The model under review builds one solid part; all positions refer to its coordinate system, in mm. Give positions to 0.01 mm unless a question says otherwise; leave off trailing zeros. Loops run counter-clockwise (first coordinate to the right, second up) from the corner with the lowest first, then second, coordinate; pieces in that order, holes last. Notation, with made-up numbers: M 11,15 L 45,15 A11 cw 45,19 Z; hole C 47.5,4.25 d2. An arc over 180 degrees is marked long. Return JSON: item names as keys, results as strings. Group by question number.
```python
from build123d import *

# Parameters (mm, degrees)
F0_R     = 3.35
F1_DEPTH = 100


with BuildPart() as f1:
    # F0 (on Top) → F1 (new body)
    with BuildSketch(Plane.XY):
        with BuildLine():
            Line((20, -15.994185), (20, -5.1))
            ThreePointArc((20, -5.1), (19.707107, -4.392893), (19, -4.1))
            Line((19, -4.1), (16.35, -4.1))
            ThreePointArc((16.35, -4.1), (15.642893, -4.392893), (15.35, -5.1))
            Line((15.35, -5.1), (15.35, -6.1))
            ThreePointArc((15.35, -6.1), (15.642893, -6.807107), (16.35, -7.1))
            Line((16.35, -7.1), (17.85, -7.1))
            ThreePointArc((17.85, -7.1), (18.203553, -7.246447), (18.35, -7.6))
            ThreePointArc((18.35, -7.6), (17.617767, -9.367767), (15.85, -10.1))
            Line((15.85, -10.1), (13.993362, -10.1))
            ThreePointArc((13.993362, -10.1), (13.036864, -9.909786), (12.225917, -9.368088))
            Line((12.225917, -9.368088), (8.332554, -5.476141))
            ThreePointArc((8.332554, -5.476141), (7.790388, -4.664971), (7.6, -3.708053))
            Line((7.6, -3.708053), (7.6, 3.708053))
            ThreePointArc((7.6, 3.708053), (7.790388, 4.664971), (8.332554, 5.476141))
            Line((8.332554, 5.476141), (12.225917, 9.368088))
            ThreePointArc((12.225917, 9.368088), (13.036864, 9.909786), (13.993362, 10.1))
            Line((13.993362, 10.1), (15.85, 10.1))
            ThreePointArc((15.85, 10.1), (17.617767, 9.367767), (18.35, 7.6))
            ThreePointArc((18.35, 7.6), (18.203553, 7.246447), (17.85, 7.1))
            Line((17.85, 7.1), (16.35, 7.1))
            ThreePointArc((16.35, 7.1), (15.642893, 6.807107), (15.35, 6.1))
            Line((15.35, 6.1), (15.35, 5.1))
            ThreePointArc((15.35, 5.1), (15.642893, 4.392893), (16.35, 4.1))
            Line((16.35, 4.1), (19, 4.1))
            ThreePointArc((19, 4.1), (19.707107, 4.392893), (20, 5.1))
            Line((20, 5.1), (20, 16.004817))
            ThreePointArc((20, 16.004817), (18.827561, 18.834111), (15.997549, 20.004817))
            Line((15.997549, 20.004817), (5.10727, 19.998145))
            ThreePointArc((5.10727, 19.998145), (4.400057, 19.705509), (4.106906, 18.998508))
            Line((4.106906, 18.998508), (4.105943, 16.348509))
            ThreePointArc((4.105943, 16.348509), (4.398579, 15.641295), (5.105579, 15.348145))
            Line((5.105579, 15.348145), (6.105579, 15.347782))
            ThreePointArc((6.105579, 15.347782), (6.812793, 15.640418), (7.105943, 16.347418))
            Line((7.105943, 16.347418), (7.106488, 17.847418))
            ThreePointArc((7.106488, 17.847418), (7.253063, 18.200918), (7.60667, 18.347236))
            ThreePointArc((7.60667, 18.347236), (9.374171, 17.614361), (10.105761, 15.846328))
            Line((10.105761, 15.846328), (10.105086, 13.98969))
            ThreePointArc((10.105086, 13.98969), (9.914524, 13.03326), (9.372532, 12.222511))
            Line((9.372532, 12.222511), (5.479169, 8.330563))
            ThreePointArc((5.479169, 8.330563), (4.667803, 7.788692), (3.710815, 7.598652))
            Line((3.710815, 7.598652), (-3.710815, 7.598652))
            ThreePointArc((-3.710815, 7.598652), (-4.667803, 7.788692), (-5.479169, 8.330563))
            Line((-5.479169, 8.330563), (-9.372532, 12.222511))
            ThreePointArc((-9.372532, 12.222511), (-9.914524, 13.03326), (-10.105086, 13.98969))
            Line((-10.105086, 13.98969), (-10.105761, 15.846328))
            ThreePointArc((-10.105761, 15.846328), (-9.374171, 17.614361), (-7.60667, 18.347236))
            ThreePointArc((-7.60667, 18.347236), (-7.253063, 18.200918), (-7.106488, 17.847418))
            Line((-7.106488, 17.847418), (-7.105943, 16.347418))
            ThreePointArc((-7.105943, 16.347418), (-6.812793, 15.640418), (-6.105579, 15.347782))
            Line((-6.105579, 15.347782), (-5.105579, 15.348145))
            ThreePointArc((-5.105579, 15.348145), (-4.398579, 15.641295), (-4.105943, 16.348509))
            Line((-4.105943, 16.348509), (-4.106906, 18.998508))
            ThreePointArc((-4.106906, 18.998508), (-4.400057, 19.705509), (-5.10727, 19.998145))
            Line((-5.10727, 19.998145), (-16.001454, 19.994185))
            ThreePointArc((-16.001454, 19.994185), (-18.828941, 18.822098), (-20, 15.994185))
            Line((-20, 15.994185), (-20, 5.1))
            ThreePointArc((-20, 5.1), (-19.707107, 4.392893), (-19, 4.1))
            Line((-19, 4.1), (-16.35, 4.1))
            ThreePointArc((-16.35, 4.1), (-15.642893, 4.392893), (-15.35, 5.1))
            Line((-15.35, 5.1), (-15.35, 6.1))
            ThreePointArc((-15.35, 6.1), (-15.642893, 6.807107), (-16.35, 7.1))
            Line((-16.35, 7.1), (-17.85, 7.1))
            ThreePointArc((-17.85, 7.1), (-18.203553, 7.246447), (-18.35, 7.6))
            ThreePointArc((-18.35, 7.6), (-17.617767, 9.367767), (-15.85, 10.1))
            Line((-15.85, 10.1), (-13.993362, 10.1))
            ThreePointArc((-13.993362, 10.1), (-13.036864, 9.909786), (-12.225917, 9.368088))
            Line((-12.225917, 9.368088), (-8.332554, 5.476141))
            ThreePointArc((-8.332554, 5.476141), (-7.790388, 4.664971), (-7.6, 3.708053))
            Line((-7.6, 3.708053), (-7.6, -3.708053))
            ThreePointArc((-7.6, -3.708053), (-7.790388, -4.664971), (-8.332554, -5.476141))
            Line((-8.332554, -5.476141), (-12.225917, -9.368088))
            ThreePointArc((-12.225917, -9.368088), (-13.036864, -9.909786), (-13.993362, -10.1))
            Line((-13.993362, -10.1), (-15.85, -10.1))
            ThreePointArc((-15.85, -10.1), (-17.617767, -9.367767), (-18.35, -7.6))
            ThreePointArc((-18.35, -7.6), (-18.203553, -7.246447), (-17.85, -7.1))
            Line((-17.85, -7.1), (-16.35, -7.1))
            ThreePointArc((-16.35, -7.1), (-15.642893, -6.807107), (-15.35, -6.1))
            Line((-15.35, -6.1), (-15.35, -5.1))
            ThreePointArc((-15.35, -5.1), (-15.642893, -4.392893), (-16.35, -4.1))
            Line((-16.35, -4.1), (-19, -4.1))
            ThreePointArc((-19, -4.1), (-19.707107, -4.392893), (-20, -5.1))
            Line((-20, -5.1), (-20, -15.994185))
            ThreePointArc((-20, -15.994185), (-18.828941, -18.822098), (-16.001454, -19.994185))
            Line((-16.001454, -19.994185), (-5.10727, -19.998145))
            ThreePointArc((-5.10727, -19.998145), (-4.400057, -19.705509), (-4.106906, -18.998508))
            Line((-4.106906, -18.998508), (-4.105943, -16.348509))
            ThreePointArc((-4.105943, -16.348509), (-4.398579, -15.641295), (-5.105579, -15.348145))
            Line((-5.105579, -15.348145), (-6.105579, -15.347782))
            ThreePointArc((-6.105579, -15.347782), (-6.812793, -15.640418), (-7.105943, -16.347418))
            Line((-7.105943, -16.347418), (-7.106488, -17.847418))
            ThreePointArc((-7.106488, -17.847418), (-7.253063, -18.200918), (-7.60667, -18.347236))
            ThreePointArc((-7.60667, -18.347236), (-9.374171, -17.614361), (-10.105761, -15.846328))
            Line((-10.105761, -15.846328), (-10.105086, -13.98969))
            ThreePointArc((-10.105086, -13.98969), (-9.914524, -13.03326), (-9.372532, -12.222511))
            Line((-9.372532, -12.222511), (-5.479169, -8.330563))
            ThreePointArc((-5.479169, -8.330563), (-4.667803, -7.788692), (-3.710815, -7.598652))
            Line((-3.710815, -7.598652), (3.710815, -7.598652))
            ThreePointArc((3.710815, -7.598652), (4.667803, -7.788692), (5.479169, -8.330563))
            Line((5.479169, -8.330563), (9.372532, -12.222511))
            ThreePointArc((9.372532, -12.222511), (9.914524, -13.03326), (10.105086, -13.98969))
            Line((10.105086, -13.98969), (10.105761, -15.846328))
            ThreePointArc((10.105761, -15.846328), (9.374171, -17.614361), (7.60667, -18.347236))
            ThreePointArc((7.60667, -18.347236), (7.253063, -18.200918), (7.106488, -17.847418))
            Line((7.106488, -17.847418), (7.105943, -16.347418))
            ThreePointArc((7.105943, -16.347418), (6.812793, -15.640418), (6.105579, -15.347782))
            Line((6.105579, -15.347782), (5.105579, -15.348145))
            ThreePointArc((5.105579, -15.348145), (4.398579, -15.641295), (4.105943, -16.348509))
            Line((4.105943, -16.348509), (4.106906, -18.998508))
            ThreePointArc((4.106906, -18.998508), (4.400057, -19.705509), (5.10727, -19.998145))
            Line((5.10727, -19.998145), (16.001454, -19.994185))
            ThreePointArc((16.001454, -19.994185), (18.828941, -18.822098), (20, -15.994185))
        make_face()
        with BuildLine():
            ThreePointArc((-16.002998, -18.346327), (-17.664699, -17.658028), (-18.352998, -15.996327))
            Line((-18.352998, -15.996327), (-18.352998, -12.544276))
            Line((-18.352998, -12.544276), (-12.548836, -12.544276))
            Line((-12.548836, -12.544276), (-12.548836, -18.346327))
            Line((-12.548836, -18.346327), (-16.002998, -18.346327))
        make_face(mode=Mode.SUBTRACT)
        with BuildLine():
            ThreePointArc((18.352998, -15.996327), (17.664699, -17.658028), (16.002998, -18.346327))
            Line((16.002998, -18.346327), (12.548836, -18.346327))
            Line((12.548836, -18.346327), (12.548836, -12.544276))
            Line((12.548836, -12.544276), (18.352998, -12.544276))
            Line((18.352998, -12.544276), (18.352998, -15.996327))
        make_face(mode=Mode.SUBTRACT)
        Circle(F0_R, mode=Mode.SUBTRACT)
        with BuildLine():
            Line((-16.002998, 18.346327), (-12.548836, 18.346327))
            Line((-12.548836, 18.346327), (-12.548836, 12.544276))
            Line((-12.548836, 12.544276), (-18.352998, 12.544276))
            Line((-18.352998, 12.544276), (-18.352998, 15.996327))
            ThreePointArc((-18.352998, 15.996327), (-17.664699, 17.658028), (-16.002998, 18.346327))
        make_face(mode=Mode.SUBTRACT)
        with BuildLine():
            Line((12.548836, 18.346327), (16.002998, 18.346327))
            ThreePointArc((16.002998, 18.346327), (17.664699, 17.658028), (18.352998, 15.996327))
            Line((18.352998, 15.996327), (18.352998, 12.544276))
            Line((18.352998, 12.544276), (12.548836, 12.544276))
            Line((12.548836, 12.544276), (12.548836, 18.346327))
        make_face(mode=Mode.SUBTRACT)
    extrude(amount=F1_DEPTH)


solid = f1.part
```
(1) Mouldability with a two-part tool opening along X and no side actions: class faces 1 (the flat face through (-2, 3, 0)), 2 (the flat face through (-7.6, 0, 49)), 3 (the flat face through (18.353, 14, 49)) as released by +X, released by -X, zero draft, split by the parting line, or undercut.
(2) Add section A-A (x = 0). Write out the cut boundary in (y, z), and give its area (3 significant figures).
(3) For probe 1 along Y at (x, z) = (5.5, 83); probe 2 along X at (y, z) = (-5.5, 50); probe 3 along Y at (x, z) = (0, 24), list the stretches that pass through material, from the lowest coordinate up.
(4) Add section C-C (z = 16.5). Count the separate pieces of the cut face and the enclosed holes in it, and give its area (3 significant figures).
(5) For pin 1 (3.5 mm diameter, centred on x = -1, z = 41.5, fed in from -Y); pin 2 (0.8 mm diameter, centred on y = 17, z = 43, fed in from -X); pin 3 (4 mm diameter, centred on x = -14, z = 71.5, fed in from -Y), all flat-tipped, find the tip position at first contact; note any pin that passes through.
Verdict:
{
 "1": {"face 1": "zero draft", "face 2": "released by -X", "face 3": "undercut"},
 "2": {"outline": "M -7.6,0 L -3.35,0 L -3.35,100 L -7.6,100 Z; M 3.35,0 L 7.6,0 L 7.6,100 L 3.35,100 Z", "area": "850 mm²"},
 "3": {"probe 1": "y = -20 to -15.35, -8.35 to 8.35, 15.35 to 20", "probe 2": "x = -20 to -15.35, -8.36 to 8.36, 15.35 to 20", "probe 3": "y = -7.6 to -3.35, 3.35 to 7.6"},
 "4": {"separate pieces": "1", "enclosed holes": "5", "area": "693 mm²"},
 "5": {"pin 1": "stops at y = -7.6", "pin 2": "stops at x = -19.95", "pin 3": "stops at y = -20"}
}
